Work out the finished part from the listing and answer in its coordinate system (mm). Face numbers are marked on the shaded views. A direction names the side the tool comes from. Coordinates: 2 decimals unless noted, no trailing zeros. Order: outer loops, then holes, each group sorted by start corner. A loop starts at its lowest first (then second) coordinate and runs counter-clockwise, first axis right, second up. Notation, with made-up numbers: M -29.75,-24 L -18.75,-24 A27 cw -18.75,-3 Z; hole C 6,30 d8. An arc over 180 degrees is marked long. Use a Markdown table: item, result.
from build123d import *

# Parameters (mm, degrees)
SKETCH1_W             = 116
SKETCH1_H             = 48.6986
BOSS_EXTRUDE1_DEPTH   = 3.175
SKETCH2_W             = 14.431210835
SKETCH2_H             = 6.35
CUT_EXTRUDE1_DEPTH    = 95.79098388
SKETCH3_W             = 14.431210835
SKETCH3_H             = 6.35
CUT_EXTRUDE2_DEPTH    = 95.79098388
SKETCH4_W             = 87.13757833
SKETCH4_H             = 3.175
BOSS_EXTRUDE2_DEPTH   = 26.9748
SKETCH5_W             = 3.678354521
SKETCH5_H             = 6.35
SKETCH6_W             = 3.671158805
SKETCH6_H             = 6.35
F_2_CLEARANCE_HOLE1_D = 2.5
F_6_CLEARANCE_HOLE1_D = 4
SKETCH11_W            = 17
SKETCH11_H            = 4
BOSS_EXTRUDE3_DEPTH   = 5.715
SKETCH12_W            = 17
SKETCH12_H            = 3.715
BOSS_EXTRUDE4_DEPTH   = 19.05
SKETCH13_R            = 2
CUT_EXTRUDE3_DEPTH    = 98.974438682
SKETCH14_W            = 35.068789165
SKETCH14_H            = 3.175
CUT_EXTRUDE4_DEPTH    = 3.175
FILLET1_R             = 12.7


with BuildPart() as part:
    # Sketch1 → Boss-Extrude1 (new body)
    with BuildSketch(Plane(origin=(0, 0, 0), x_dir=(-1, 0, 0), z_dir=(0, 0, -1))):
        with Locations((29, -13.1507)):
            Rectangle(SKETCH1_W, SKETCH1_H)
    extrude(amount=-BOSS_EXTRUDE1_DEPTH)

    # Sketch2 → Cut-Extrude1 (cut, through all)
    with BuildSketch(Plane.XY.offset(3.175)):
        with Locations((21.784394583, 8.0236)):
            Rectangle(SKETCH2_W, SKETCH2_H)
    extrude(amount=-CUT_EXTRUDE1_DEPTH, mode=Mode.SUBTRACT)

    # Sketch3 → Cut-Extrude2 (cut, through all)
    with BuildSketch(Plane.XY.offset(3.175)):
        with Locations((-79.784394582, 8.0236)):
            Rectangle(SKETCH3_W, SKETCH3_H)
    extrude(amount=-CUT_EXTRUDE2_DEPTH, mode=Mode.SUBTRACT)

    # Sketch4 → Boss-Extrude2 (add)
    with BuildSketch(Plane(origin=(0, 0, 0), x_dir=(-1, 0, 0), z_dir=(0, 0, -1))):
        with Locations((29, 9.6111)):
            Rectangle(SKETCH4_W, SKETCH4_H)
    extrude(amount=BOSS_EXTRUDE2_DEPTH)

    # Sketch5 → Revolve1 (revolve)
    with BuildSketch(Plane(origin=(0, 0, -14.77), x_dir=(-1, 0, 0), z_dir=(0, 0, -1)), mode=Mode.PRIVATE) as revolve1_sk:
        with Locations((-11.889177261, 4.8486)):
            Rectangle(SKETCH5_W, SKETCH5_H)
    revolve(revolve1_sk.sketch.rotate(Axis((10.05, 1.6736, -14.77), (0, 1, 0)), 270), axis=Axis((10.05, 1.6736, -14.77), (0, 1, 0)))

    # Sketch6 → Revolve2 (revolve)
    with BuildSketch(Plane(origin=(0, 0, -14.97), x_dir=(-1, 0, 0), z_dir=(0, 0, -1)), mode=Mode.PRIVATE) as revolve2_sk:
        with Locations((66.214420598, 4.8486)):
            Rectangle(SKETCH6_W, SKETCH6_H)
    revolve(revolve2_sk.sketch.rotate(Axis((-68.05, 1.6736, -14.97), (0, 1, 0)), 270), axis=Axis((-68.05, 1.6736, -14.97), (0, 1, 0)))

    # #2 Clearance Hole1 (through all)
    with Locations(Plane(origin=(0, 0, 0), x_dir=(-1, 0, 0), z_dir=(0, 0, -1))):
        with Locations((72.699747468, -30.449747468), (65, -12.13), (51, -12.13), (43.300252532, -30.449747468), (14.699747468, -30.449747468), (7, -12.13), (-7, -12.13), (-14.699747468, -30.449747468)):
            Hole(F_2_CLEARANCE_HOLE1_D / 2)

    # #6 Clearance Hole1 (through all)
    with Locations(Plane(origin=(0, 0, 0), x_dir=(-1, 0, 0), z_dir=(0, 0, -1))):
        with Locations((33.75, -22.13), (82.25, -12.13), (82.25, -22.13), (-24.25, -12.13), (24.25, -12.13), (24.25, -22.13), (33.75, -12.13), (-24.25, -22.13)):
            Hole(F_6_CLEARANCE_HOLE1_D / 2)

    # Sketch11 → Boss-Extrude3 (add)
    with BuildSketch(Plane(origin=(0, 0, 0), x_dir=(-1, 0, 0), z_dir=(0, 0, -1))):
        with Locations((29, -5)):
            Rectangle(SKETCH11_W, SKETCH11_H)
    extrude(amount=BOSS_EXTRUDE3_DEPTH)

    # Sketch12 → Boss-Extrude4 (add)
    with BuildSketch(Plane.XZ.offset(7)):
        with Locations((-29, -3.8575)):
            Rectangle(SKETCH12_W, SKETCH12_H)
    extrude(amount=BOSS_EXTRUDE4_DEPTH)

    # Sketch13 → Cut-Extrude3 (cut, through all)
    with BuildSketch(Plane.XY.offset(-2)):
        with Locations(Location((-33.75, -12.13, 0), (0, 0, 180))):
            Circle(SKETCH13_R)
        with Locations(Location((-24.25, -12.13, 0), (0, 0, 180))):
            Circle(SKETCH13_R)
        with Locations(Location((-24.25, -22.13, 0), (0, 0, 180))):
            Circle(SKETCH13_R)
        with Locations(Location((-33.75, -22.13, 0), (0, 0, 180))):
            Circle(SKETCH13_R)
    extrude(amount=-CUT_EXTRUDE3_DEPTH, mode=Mode.SUBTRACT)

    # Sketch14 → Cut-Extrude4 (cut)
    with BuildSketch(Plane(origin=(0, 0, 0), x_dir=(-1, 0, 0), z_dir=(0, 0, -1))):
        with Locations((2.965605417, 6.4361)):
            Rectangle(SKETCH14_W, SKETCH14_H)
        with Locations((55.034394582, 6.4361)):
            Rectangle(SKETCH14_W, SKETCH14_H)
    extrude(amount=-CUT_EXTRUDE4_DEPTH, mode=Mode.SUBTRACT)

    # Fillet1
    fillet1_edges = [part.edges().sort_by_distance(p)[0] for p in [
        (29, 4.8486, 1.5875),
        (14.568789165, 9.6111, 3.175),
        (-72.568789165, 9.6111, 3.175),
        (-87, 4.8486, 1.5875),
        (-72.568789165, 9.6111, -26.9748),
        (14.568789165, 9.6111, -26.9748),
        (29, -37.5, 1.5875),
        (-87, -37.5, 1.5875),
    ]]
    fillet(fillet1_edges, radius=FILLET1_R)


solid = part.part
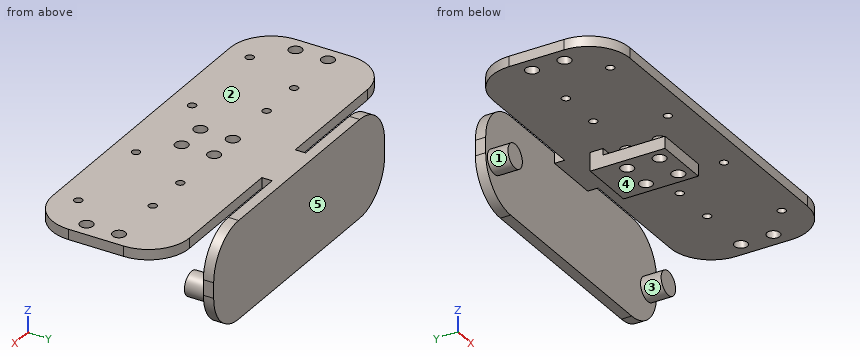
(1) Given P1, Ø3, axis at x = 24.25, y = -22.13, coming from the -Z side; P2, Ø6.5, axis at y = -20, z = -3.5, coming from the -X side; P3, Ø12, axis at x = -59.5, z = -14, coming from the -Y side; P4, Ø4, axis at x = 14.7, y = -30.45, coming from the -Z side, each flat-ended and moving along its own axis, determine where each tip first touches the part or whether it passes through.
Conclusion:
| item | result |
|---|---|
| P1 | through |
| P2 | x = -37.5 |
| P3 | y = 1.67 |
| P4 | z = 0 |
(2) Determine the mould class of the marked faces 1, 2 and 3 for opening direction X: pulls with the +X half, pulls with the -X half, needs draft (parallel to the pull), parting line crosses it, or undercut.
Conclusion:
| item | result |
|---|---|
| face 1 | undercut |
| face 2 | needs draft |
| face 3 | undercut |
(3) A cutting plane is placed at B-B (y = -22.13). Give the number of separate pieces and of enclosed holes in the cut face, then the cut area to 3 significant figures.
Conclusion:
| item | result |
|---|---|
| separate pieces | 8 |
| enclosed holes | 0 |
| area | 351 mm2 |
(4) Which of the six approach directions +Z, -Z, +X, -X, +Y, -Y give full straight-line access (tool end or side, diameter ignored) to the marked faces 4 and 5?
Conclusion:
| item | result |
|---|---|
| face 4 | -Z, +X, -X, -Y |
| face 5 | +Z, -Z, +X, -X, +Y |
(5) Straight lines are drawn through the part: L1, parallel to X at y = -22, z = 2; L2, parallel to Y at x = -7, z = 1; L3, parallel to X at y = -12.13, z = -4.7. For each, find the intervals that lie inside material, in ascending order.
Conclusion:
| item | result |
|---|---|
| L1 | -87 to -84.25, -80.25 to -35.75, -31.75 to -26.25, -22.25 to 22.25, 26.25 to 29 |
| L2 | -37.5 to -13.38, -10.88 to 4.85, 8.02 to 11.2 |
| L3 | -37.5 to -35.75, -31.75 to -26.25, -22.25 to -20.5 |
(6) A cutting plane is placed at D-D (x = -68.05). Determine the outline of the cut face in (y, z) (3 decimals), then the cut area to 3 significant figures.
Conclusion:
| item | result |
|---|---|
| outline | M -37.5,0 L 4.849,0 L 4.849,3.175 L -37.5,3.175 Z; M 1.674,-18.641 L 8.024,-18.641 L 8.024,-23.989 L 11.199,-23.989 L 11.199,0.189 L 8.024,0.189 L 8.024,-11.299 L 1.674,-11.299 Z |
| area | 258 mm2 |
(7) A cutting plane is placed at C-C (x = -24.25). Determine the outline of the cut face in (y, z) (3 decimals), then the cut area to 3 significant figures.
Conclusion:
| item | result |
|---|---|
| outline | M -37.5,0 L -24.13,0 L -24.13,3.175 L -37.5,3.175 Z; M -26.05,-5.715 L -24.13,-5.715 L -24.13,-2 L -26.05,-2 Z; M -20.13,-5.715 L -14.13,-5.715 L -14.13,-2 L -20.13,-2 Z; M -20.13,0 L -14.13,0 L -14.13,3.175 L -20.13,3.175 Z; M -10.13,-5.715 L -3,-5.715 L -3,0 L 8.024,0 L 8.024,-26.975 L 11.199,-26.975 L 11.199,3.175 L -10.13,3.175 L -10.13,0 L -7,0 L -7,-2 L -10.13,-2 Z |
| area | 279 mm2 |
(8) A cutting plane is placed at A-A (x = -51). Determine the outline of the cut face in (y, z) (3 decimals), then the cut area to 3 significant figures.
Conclusion:
| item | result |
|---|---|
| outline | M -37.5,0 L -13.38,0 L -13.38,3.175 L -37.5,3.175 Z; M -10.88,0 L 4.849,0 L 4.849,3.175 L -10.88,3.175 Z; M 8.024,-26.975 L 11.199,-26.975 L 11.199,3.175 L 8.024,3.175 Z |
| area | 222 mm2 |
